from build123d import *

# Parameters (mm, degrees)
F0_W     = 15.24
F0_H     = 38.1
F0_W_2   = 7.112
F0_H_2   = 19.05
F1_DEPTH = 3.175
F2_W     = 12.7
F2_H     = 31.75
F2_W_2   = 7.112
F2_H_2   = 19.05
F3_DEPTH = 1.905
F0_H_3   = 3.175
F4_DEPTH = 12.7


with BuildPart() as f1:
    # F0 (on Top) → F1 (new body)
    with BuildSketch(Plane.XY):
        with Locations((7.62, 19.05)):
            Rectangle(F0_W, F0_H)
        with Locations((7.366, 19.685)):
            Rectangle(F0_W_2, F0_H_2, mode=Mode.SUBTRACT)
    extrude(amount=F1_DEPTH)

    # F2 (on face) → F3 (cut)
    with BuildSketch(Plane.XY.offset(3.175)):
        with Locations((7.62, 19.685)):
            Rectangle(F2_W, F2_H)
        with Locations((7.366, 19.685)):
            Rectangle(F2_W_2, F2_H_2, mode=Mode.SUBTRACT)
    extrude(amount=-F3_DEPTH, mode=Mode.SUBTRACT)

    # F0 (on Top) → F4 (join)
    with BuildSketch(Plane.XY):
        with Locations((7.62, -1.5875)):
            Rectangle(F0_W, F0_H_3)
    extrude(amount=F4_DEPTH)


solid = f1.part
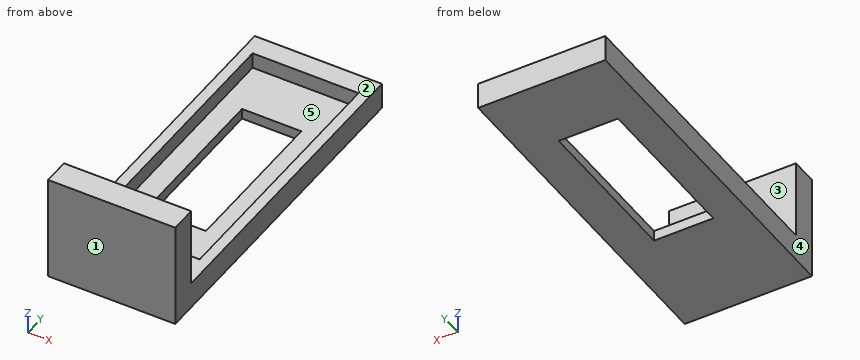
CAD build for the part. Positions are in the model's coordinates, mm. Face numbers are marked on the shaded views. A direction names the side the tool comes from. Coordinates: 2 decimals unless noted, no trailing zeros. Loops run counter-clockwise (first coordinate to the right, second up) from the corner with the lowest first, then second, coordinate; pieces in that order, holes last. Notation, with made-up numbers: (-36.75, 84) -> (-0.75, 84) arc R14 ccw to (-0.75, 104) -> close; hole circle Ø7 at (30, 68). An arc over 180 degrees is marked (long way). One line per item, written item: value.
1. Which spindle directions (+Z, -Z, +X, -X, +Y, -Y) get a long thin tool onto all of the face, cutting with end or side? Do the marked faces 1 and 2. Say none if no direction does.
Answers:
face 1: +Z, -Z, +X, -X, -Y
face 2: +Z, +X, -X, +Y
2. Slice it at C-C on x = 5.5. Write the cut outline in (y, z) (3 decimals).
Answers:
outline: (-3.175, 0) -> (10.16, 0) -> (10.16, 1.27) -> (3.81, 1.27) -> (3.81, 3.175) -> (0, 3.175) -> (0, 12.7) -> (-3.175, 12.7) -> close; (29.21, 0) -> (38.1, 0) -> (38.1, 3.175) -> (35.56, 3.175) -> (35.56, 1.27) -> (29.21, 1.27) -> close
3. Flat gauge pins, fed straight in: P1, Ø3, axis at x = 5.5, y = 32, coming from the +Z side; P2, Ø1.5, axis at x = 6.5, y = 25.5, coming from the -Z side; P3, Ø1.5, axis at x = 13.5, z = 5.5, coming from the +Y side. Where does each tip first touch, or does it go through?
Answers:
P1: stops at z = 1.27
P2: passes through
P3: stops at y = 0
4. Slice it at B-B on z = 1.75. Write the cut outline in (x, y) (3 decimals), and give its area (3 significant figures).
Answers:
outline: (0, -3.175) -> (15.24, -3.175) -> (15.24, 38.1) -> (0, 38.1) -> close; hole (1.27, 3.81) -> (13.97, 3.81) -> (13.97, 35.56) -> (1.27, 35.56) -> close
area: 226 mm^2
5. Drill centre lines: line 1 (X direction, y = 35, z = 1.75); line 2 (Y direction, x = 10, z = 6) (3 decimals); line 3 (Z direction, x = 4.5, y = 1) (3 decimals). Where is each one in solid material? Low to high. Write a range as [from, to].
Answers:
line 1: x = [0, 1.27], [13.97, 15.24]
line 2: y = [-3.175, 0]
line 3: z = [0, 3.175]
6. Slice it at D-D on x = 2. Write the cut outline in (y, z) (3 decimals), and give its area (3 significant figures).
Answers:
outline: (-3.175, 0) -> (38.1, 0) -> (38.1, 3.175) -> (35.56, 3.175) -> (35.56, 1.27) -> (3.81, 1.27) -> (3.81, 3.175) -> (0, 3.175) -> (0, 12.7) -> (-3.175, 12.7) -> close
area: 101 mm^2
7. Slice it at A-A on y = 27.5. Write the cut outline in (x, z) (3 decimals).
Answers:
outline: (0, 0) -> (3.81, 0) -> (3.81, 1.27) -> (1.27, 1.27) -> (1.27, 3.175) -> (0, 3.175) -> close; (10.922, 0) -> (15.24, 0) -> (15.24, 3.175) -> (13.97, 3.175) -> (13.97, 1.27) -> (10.922, 1.27) -> close
8. Pull direction X, two halves, no side cores. Call the marked faces 3, 4 and 5: pulls with the +X half, pulls with the -X half, needs draft (parallel to the pull), parting line crosses it, or undercut.
Answers:
face 3: needs draft
face 4: pulls with the -X half
face 5: undercut
